Design review of the part built by this model. Coordinates are the model's own, in mm. A direction names the side the tool comes from. Round coordinates to 2 decimals unless told otherwise and drop trailing zeros. Order: outer loops, then holes, each group sorted by start corner. A loop starts at its lowest first (then second) coordinate and runs counter-clockwise, first axis right, second up.
from build123d import *

# Parameters (mm, degrees)
SKETCH1_R           = 2.75
SKETCH1_R_2         = 2
BOSS_EXTRUDE1_DEPTH = 3


with BuildPart() as part:
    # Sketch1 → Boss-Extrude1 (new body)
    with BuildSketch(Plane(origin=(0, 0, 0), x_dir=(0, 1, 0), z_dir=(0, 0, 1))):
        with BuildLine():
            Line((-16.064138017, 18.25), (-11.5, 18.25))
            ThreePointArc((-11.5, 18.25), (-11.146446609, 18.103553391), (-11, 17.75))
            Line((-11, 17.75), (-11, 15.883140649))
            ThreePointArc((-11, 15.883140649), (-11.240562739, 15.455715442), (-11.730769231, 15.439580549))
            ThreePointArc((-11.730769231, 15.439580549), (-15.75, 13), (-11.730769231, 10.560419451))
            ThreePointArc((-11.730769231, 10.560419451), (-11.240562739, 10.544284558), (-11, 10.116859351))
            Line((-11, 10.116859351), (-11, 0))
            ThreePointArc((-11, 0), (0, -11), (11, 0))
            Line((11, 0), (11, 10.116859351))
            ThreePointArc((11, 10.116859351), (11.240562739, 10.544284558), (11.730769231, 10.560419451))
            ThreePointArc((11.730769231, 10.560419451), (15.75, 13), (11.730769231, 15.439580549))
            ThreePointArc((11.730769231, 15.439580549), (11.240562739, 15.455715442), (11, 15.883140649))
            Line((11, 15.883140649), (11, 17.75))
            ThreePointArc((11, 17.75), (11.146446609, 18.103553391), (11.5, 18.25))
            Line((11.5, 18.25), (16.064138017, 18.25))
            ThreePointArc((16.064138017, 18.25), (17.830790051, 17.674652674), (18.919816403, 16.169293727))
            Line((18.919816403, 16.169293727), (29.855678386, -17.801681794))
            ThreePointArc((29.855678386, -17.801681794), (29.963699981, -18.255698807), (30, -18.720975521))
            Line((30, -18.720975521), (30, -38.25))
            ThreePointArc((30, -38.25), (29.853553391, -38.603553391), (29.5, -38.75))
            Line((29.5, -38.75), (20.75, -38.75))
            ThreePointArc((20.75, -38.75), (20.396446609, -38.603553391), (20.25, -38.25))
            Line((20.25, -38.25), (20.25, -19.65))
            ThreePointArc((20.25, -19.65), (19.957106781, -18.942893219), (19.25, -18.65))
            Line((19.25, -18.65), (-19.25, -18.65))
            ThreePointArc((-19.25, -18.65), (-19.957106781, -18.942893219), (-20.25, -19.65))
            Line((-20.25, -19.65), (-20.25, -38.25))
            ThreePointArc((-20.25, -38.25), (-20.396446609, -38.603553391), (-20.75, -38.75))
            Line((-20.75, -38.75), (-29.5, -38.75))
            ThreePointArc((-29.5, -38.75), (-29.853553391, -38.603553391), (-30, -38.25))
            Line((-30, -38.25), (-30, -18.720975521))
            ThreePointArc((-30, -18.720975521), (-29.963699981, -18.255698807), (-29.855678386, -17.801681794))
            Line((-29.855678386, -17.801681794), (-18.919816403, 16.169293727))
            ThreePointArc((-18.919816403, 16.169293727), (-17.830790051, 17.674652674), (-16.064138017, 18.25))
        make_face()
        with Locations(Location((13, -13, 0), (0, 0, 270))):
            Circle(SKETCH1_R, mode=Mode.SUBTRACT)
        with Locations(Location((-13, -13, 0), (0, 0, 270))):
            Circle(SKETCH1_R, mode=Mode.SUBTRACT)
        with Locations(Location((-23.5, -23.65, 0), (0, 0, 270))):
            Circle(SKETCH1_R_2, mode=Mode.SUBTRACT)
        with Locations(Location((23.5, -23.65, 0), (0, 0, 270))):
            Circle(SKETCH1_R_2, mode=Mode.SUBTRACT)
        with Locations(Location((23.5, -33.65, 0), (0, 0, 270))):
            Circle(SKETCH1_R_2, mode=Mode.SUBTRACT)
        with Locations(Location((-23.5, -33.65, 0), (0, 0, 270))):
            Circle(SKETCH1_R_2, mode=Mode.SUBTRACT)
    extrude(amount=BOSS_EXTRUDE1_DEPTH)


solid = part.part
1) Clearance check with flat-ended pins moving along their axes: P1, Ø1.5, axis at x = -3.5, z = 2, coming from the -Y side; P2, Ø3, axis at x = 33.65, y = 23.5, coming from the -Z side; P3, Ø0.9, axis at x = -4, z = 2, coming from the +Y side; P4, Ø1.5, axis at y = 19, z = 2, coming from the -X side. State where each tip first meets the part, or that it passes through.
Results:
P1: stops at y = -23.24
P2: passes through
P3: stops at y = 22.98
P4: stops at x = -17.3
2) Take a section at D-D on x = 24.5. Give the boundary of the cut face in (y, z), plus the area to 3 significant figures.
Results:
outline: (-30, 0) - (-25.31, 0) - (-25.31, 3) - (-30, 3) - close; (-21.69, 0) - (-20.25, 0) - (-20.25, 3) - (-21.69, 3) - close; (20.25, 0) - (21.69, 0) - (21.69, 3) - (20.25, 3) - close; (25.31, 0) - (30, 0) - (30, 3) - (25.31, 3) - close
area: 36.8 mm2
3) The part is to be moulded in two halves that separate along Y. For faces 1 (the face through (1.054, -24.464, 1.479)), 2 (the face through (-17.69, 17.81, 1.48)), 3 (the face through (38.75, -25, 1)), 4 (the face through (18.65, 0, 1)), say which applies: released by +Y, released by -Y, zero draft, split by the parting line, or undercut.
Results:
face 1: released by -Y
face 2: released by +Y
face 3: zero draft
face 4: undercut
4) For faces 5 (the face through (-17, -11, 1)), 6 (the face through (25.558, -22.899, 1.479)), 7 (the face through (29, 20.25, 1)), list the 3-axis set-ups (+Z, -Z, +X, -X, +Y, -Y) from which the entire face can be reached by the end or side of a thin tool; tool diameter is ignored.
Results:
face 5: +Z, -Z, -X
face 6: +Z, -Z
face 7: +Z, -Z, +X
5) To check wall thickness, follow line 1 along Y through (x, z) = (23.65, 0.8); line 2 along Y through (x, z) = (25, 2.4); line 3 along Y through (x, z) = (12, 1.9). State the ranges of each line that lie inside material, in increasing order.
Results:
line 1: y = -30 to -25.5, -21.5 to -20.25, 20.25 to 21.5, 25.5 to 30
line 2: y = -30 to -24.98, -22.02 to -20.25, 20.25 to 22.02, 24.98 to 30
line 3: y = -27.99 to -15.56, -10.44 to 10.44, 15.56 to 27.99
6) Take a section at C-C on x = 13. Give the boundary of the cut face in (y, z), plus the area to 3 significant figures.
Results:
outline: (-28.31, 0) - (-15.75, 0) - (-15.75, 3) - (-28.31, 3) - close; (-10.25, 0) - (10.25, 0) - (10.25, 3) - (-10.25, 3) - close; (15.75, 0) - (28.31, 0) - (28.31, 3) - (15.75, 3) - close
area: 137 mm2
7) Take a section at B-B on x = -13. Give the boundary of the cut face in (y, z).
Results:
outline: (-19.94, 0) - (-15.75, 0) - (-15.75, 3) - (-19.94, 3) - close; (15.75, 0) - (19.94, 0) - (19.94, 3) - (15.75, 3) - close
8) Take a section at A-A on y = -13. Give the boundary of the cut face in (x, z), plus the area to 3 significant figures.
Results:
outline: (-18.25, 0) - (-15.75, 0) - (-15.75, 3) - (-18.25, 3) - close; (-10.25, 0) - (10.25, 0) - (10.25, 3) - (-10.25, 3) - close; (15.75, 0) - (18.65, 0) - (18.65, 3) - (15.75, 3) - close
area: 77.7 mm2
